CAD build for the part. Positions are in the model's coordinates, mm. A direction names the side the tool comes from. Round coordinates to 2 decimals unless told otherwise and drop trailing zeros. Order: outer loops, then holes, each group sorted by start corner. A loop starts at its lowest first (then second) coordinate and runs counter-clockwise, first axis right, second up. Notation, with made-up numbers: M 13,7 L 17,7 A20 ccw 17,35 Z; hole C 22.25,-28 d3. An arc over 180 degrees is marked long. Answer as a JSON object with one key per item and string values. Group by question number.
```python
from build123d import *

# Parameters (mm, degrees)
SKETCH1_R           = 6.25
SKETCH1_R_2         = 5.75
BOSS_EXTRUDE1_DEPTH = 5
SKETCH1_3_R         = 6.75
SKETCH1_3_R_2       = 6.25
BOSS_EXTRUDE2_DEPTH = 0.5


with BuildPart() as part:
    # Sketch1 → Boss-Extrude1 (new body)
    with BuildSketch(Plane(origin=(0, 0, 0), x_dir=(1, 0, 0), z_dir=(0, 1, 0))):
        with Locations(Location((0, 0, 0), (0, 0, 270))):
            Circle(SKETCH1_R)
        with Locations(Location((0, 0, 0), (0, 0, 270))):
            Circle(SKETCH1_R_2, mode=Mode.SUBTRACT)
    boss_extrude1 = extrude(amount=BOSS_EXTRUDE1_DEPTH)

    # Sketch1_3 → Boss-Extrude2 (add)
    with BuildSketch(Plane(origin=(0, 0, 0), x_dir=(1, 0, 0), z_dir=(0, 1, 0))):
        with Locations(Location((0, 0, 0), (0, 0, 270))):
            Circle(SKETCH1_3_R)
        with Locations(Location((0, 0, 0), (0, 0, 270))):
            Circle(SKETCH1_3_R_2, mode=Mode.SUBTRACT)
    boss_extrude2 = extrude(amount=BOSS_EXTRUDE2_DEPTH)

    # Mirror1: Boss-Extrude1, Boss-Extrude2 across plane
    add(boss_extrude1.mirror(Plane.ZX.offset(5)))
    add(boss_extrude2.mirror(Plane.ZX.offset(5)))


solid = part.part
```
Item 1: Cut at B-B, the plane x = -1.25. Give the cut face in (y, z).
Item 2: Cut at C-C, the plane y = 2. Give the cut face in (x, z).
Item 3: Flat gauge pins, fed straight in: pin 1 Ø2 at (x, y) = (-1, 3) entering from +Z; pin 2 Ø7 at (x, z) = (3, -1) entering from -Y; pin 3 Ø2 at (x, z) = (1.5, -3.5) entering from -Y. Where does each tip first touch, or does it go through?
Item 4: 3-axis set-ups, long thin cutter, end or side, ignore diameter. For faces 1 (the face through (-6.59, 0.25, -1.46)), 2 (the face through (1.88, 5.06, 5.96)): which of +Z, -Z, +X, -X, +Y, -Y reach the whole face in a straight line?
Item 5: Cut at A-A, the plane z = 0. Give the cut face in (x, y).
Item 6: Drill centre lines: line 1 (X direction, y = 6.25, z = 0); line 2 (Z direction, x = -2, y = 9.25); line 3 (X direction, y = 6, z = 4.5). Where is each one in solid material? Low to high. Write a range as [from, to].
Item 7: Two-plate mould, pull along X, no slides. Class faces 3 (the face through (-6.59, 9.75, -1.46)), 4 (the face through (4.85, 5.07, 3.09)), 5 (the face through (-4, 0.5, 5)): +X half, -X half, draft (parallel to the pull), parting line (faces both ways), or undercut.
Response values:
{
 "1": {"outline": "M 0,-6.63 L 0.5,-6.63 L 0.5,-6.12 L 9.5,-6.12 L 9.5,-6.63 L 10,-6.63 L 10,-5.61 L 0,-5.61 Z; M 0,5.61 L 10,5.61 L 10,6.63 L 9.5,6.63 L 9.5,6.12 L 0.5,6.12 L 0.5,6.63 L 0,6.63 Z"},
 "2": {"outline": "C 0,0 d12.5; hole C 0,0 d11.5"},
 "3": {"pin 1": "z = 6.25", "pin 2": "y = 0", "pin 3": "through"},
 "4": {"face 1": "+Y, -Y", "face 2": "none"},
 "5": {"outline": "M -6.75,0 L -5.75,0 L -5.75,10 L -6.75,10 L -6.75,9.5 L -6.25,9.5 L -6.25,0.5 L -6.75,0.5 Z; M 5.75,0 L 6.75,0 L 6.75,0.5 L 6.25,0.5 L 6.25,9.5 L 6.75,9.5 L 6.75,10 L 5.75,10 Z"},
 "6": {"line 1": "[-6.25, -5.75], [5.75, 6.25]", "line 2": "[-5.92, -5.39], [5.39, 5.92]", "line 3": "[-4.34, -3.58], [3.58, 4.34]"},
 "7": {"face 3": "parting line", "face 4": "undercut", "face 5": "draft"}
}
